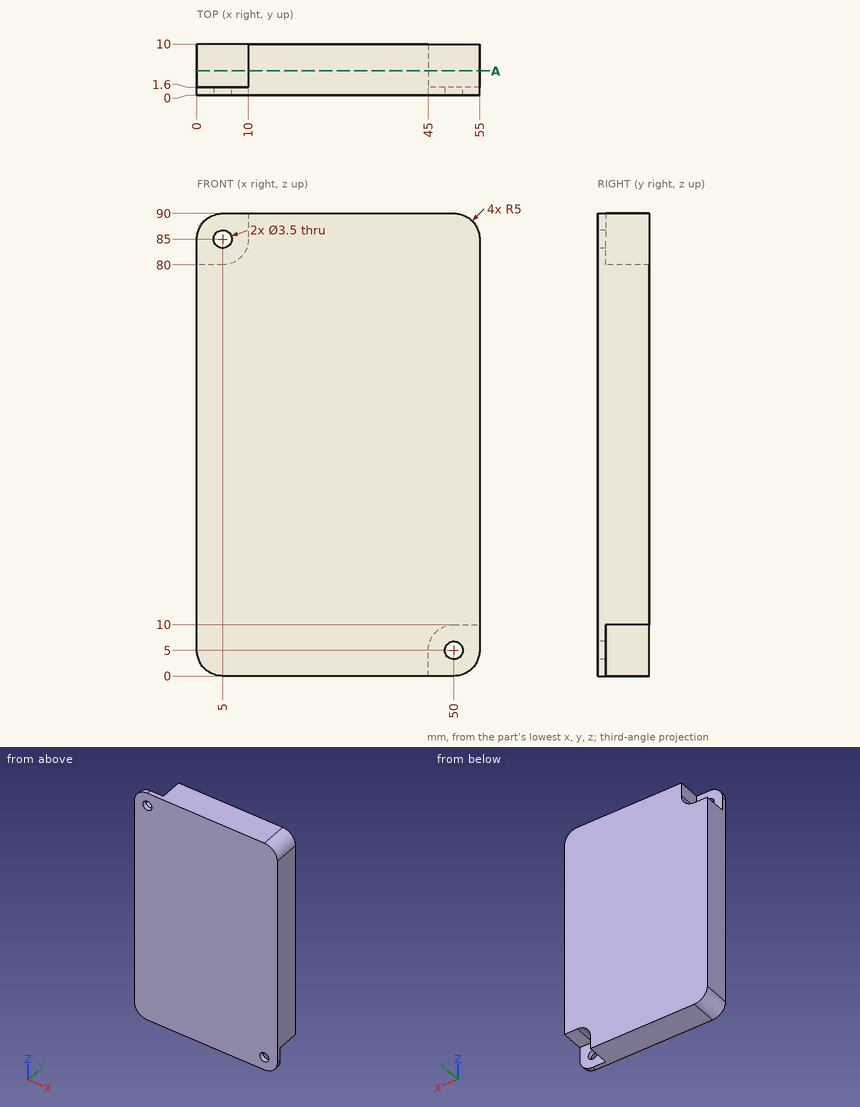
Verification items for this drawing (mm, ordinates from the low corner). Coordinates: 2 decimals unless noted, no trailing zeros. Loops run counter-clockwise (first coordinate to the right, second up) from the corner with the lowest first, then second, coordinate; pieces in that order, holes last.
Item 1: Thickness scan on line 1 (X direction, y = 1.05, z = 5); line 2 (Z direction, x = 50, y = 0.6); line 3 (X direction, y = 1.1, z = 85). Record the ranges inside material, lowest first.
Item 2: Go/stop test with flat-tipped pins: pin 1 Ø5.5 at (x, z) = (50, 5) entering from +Y; pin 2 Ø5.5 at (x, y) = (52, 5.5) entering from -Z; pin 3 Ø5.5 at (y, z) = (5.5, 88.5) entering from -X. Record where each tip stops, or that it passes through.
Item 3: Sectioned sample at A-A, the plane y = 4.75. Record the boundary of the cut face in (x, z), then the cut area to 3 significant figures.
Check result:
1. line 1: x = 0 to 48.25, 51.75 to 55
1. line 2: z = 0 to 3.25, 6.75 to 90
1. line 3: x = 0 to 3.25, 6.75 to 55
2. pin 1: stops at y = 1.6
2. pin 2: stops at z = 9.94
2. pin 3: stops at x = 10
3. outline: (0, 5) arc R5 ccw to (5, 0) - (45, 0) - (45, 5) arc R5 cw to (50, 10) - (55, 10) - (55, 85) arc R5 ccw to (50, 90) - (10, 90) - (10, 85) arc R5 cw to (5, 80) - (0, 80) - close
3. area: 4,750 mm2
